```python
from build123d import *

# Parameters (mm, degrees)
SKETCH1_W                    = 98
SKETCH1_H                    = 32.71
BASE_FLANGE1_DEPTH           = 1.016
EDGE_FLANGE1_DEPTH           = 18
EDGE_FLANGE2_STRIP_CUT_DEPTH = 98
EDGE_FLANGE2_DEPTH           = 98
EDGE_FLANGE3_STRIP_CUT_DEPTH = 98
EDGE_FLANGE3_DEPTH           = 98
CUT_EXTRUDE1_REACH           = 115.066
SKETCH17_R                   = 1.1303


# Sheet-metal steps are written as plain solids
with BuildPart() as part:
    # Sketch1 → Base-Flange1 (new body)
    with BuildSketch(Plane.XY):
        with Locations((49, 16.355)):
            Rectangle(SKETCH1_W, SKETCH1_H)
        with BuildLine():
            Line((61.25, 18.71), (61.25, 3.21))
            ThreePointArc((61.25, 3.21), (61.542893219, 2.502893219), (62.25, 2.21))
            Line((62.25, 2.21), (70.25, 2.21))
            ThreePointArc((70.25, 2.21), (70.957106781, 2.502893219), (71.25, 3.21))
            Line((71.25, 3.21), (71.25, 6.21))
            ThreePointArc((71.25, 6.21), (71.542893219, 6.917106781), (72.25, 7.21))
            Line((72.25, 7.21), (82.25, 7.21))
            ThreePointArc((82.25, 7.21), (82.957106781, 7.502893219), (83.25, 8.21))
            Line((83.25, 8.21), (83.25, 29.21))
            ThreePointArc((83.25, 29.21), (82.957106781, 29.917106781), (82.25, 30.21))
            Line((82.25, 30.21), (72.25, 30.21))
            ThreePointArc((72.25, 30.21), (71.542893219, 29.917106781), (71.25, 29.21))
            Line((71.25, 29.21), (71.25, 20.71))
            ThreePointArc((71.25, 20.71), (70.957106781, 20.002893219), (70.25, 19.71))
            Line((70.25, 19.71), (62.25, 19.71))
            ThreePointArc((62.25, 19.71), (61.542893219, 19.417106781), (61.25, 18.71))
        make_face(mode=Mode.SUBTRACT)
        with BuildLine():
            Line((25.75, 30.21), (15.75, 30.21))
            ThreePointArc((15.75, 30.21), (15.042893219, 29.917106781), (14.75, 29.21))
            Line((14.75, 29.21), (14.75, 8.21))
            ThreePointArc((14.75, 8.21), (15.042893219, 7.502893219), (15.75, 7.21))
            Line((15.75, 7.21), (25.75, 7.21))
            ThreePointArc((25.75, 7.21), (26.457106781, 6.917106781), (26.75, 6.21))
            Line((26.75, 6.21), (26.75, 3.21))
            ThreePointArc((26.75, 3.21), (27.042893219, 2.502893219), (27.75, 2.21))
            Line((27.75, 2.21), (35.75, 2.21))
            ThreePointArc((35.75, 2.21), (36.457106781, 2.502893219), (36.75, 3.21))
            Line((36.75, 3.21), (36.75, 18.71))
            ThreePointArc((36.75, 18.71), (36.457106781, 19.417106781), (35.75, 19.71))
            Line((35.75, 19.71), (27.75, 19.71))
            ThreePointArc((27.75, 19.71), (27.042893219, 20.002893219), (26.75, 20.71))
            Line((26.75, 20.71), (26.75, 29.21))
            ThreePointArc((26.75, 29.21), (26.457106781, 29.917106781), (25.75, 30.21))
        make_face(mode=Mode.SUBTRACT)
    extrude(amount=-BASE_FLANGE1_DEPTH)

    # Edge-Flange1 section (across the edge) → Edge-Flange1 (add)
    with BuildSketch(Plane(origin=(40, 33.4466, -1.016), x_dir=(0, -1, 0), z_dir=(1, 0, 0))):
        with BuildLine():
            Line((-1.016, 0.7366), (-1.016, 17.984))
            Line((-1.016, 17.984), (0, 17.984))
            Line((0, 17.984), (0, 0.7366))
            ThreePointArc((0, 0.7366), (0.215745145, 0.215745145), (0.7366, 0))
            Line((0.7366, 0), (0.7366, -1.016))
            ThreePointArc((0.7366, -1.016), (-0.502675345, -0.502675345), (-1.016, 0.7366))
        make_face()
    extrude(amount=EDGE_FLANGE1_DEPTH)

    # Edge-Flange2 strip (across the edge) → Edge-Flange2 strip cut (cut)
    with BuildSketch(Plane(origin=(0, 0, 0), x_dir=(0, 0.8660254037844364, 0.5000000000000041), z_dir=(1, 0, 0))):
        Polygon((-4.935055866, 1.676080086), (-0.1397, -1.092519914), (0.3683, -0.212638104), (-4.427055866, 2.555961896), align=None)
    extrude(amount=EDGE_FLANGE2_STRIP_CUT_DEPTH, mode=Mode.SUBTRACT)

    # Edge-Flange2 section (across the edge) → Edge-Flange2 (add)
    with BuildSketch(Plane(origin=(0, 0, 0), x_dir=(0, 0.8660254037844364, 0.5000000000000041), z_dir=(1, 0, 0))):
        with BuildLine():
            Line((-1.016, 0.425276208), (-1.016, 14.163412127))
            Line((-1.016, 14.163412127), (0, 14.163412127))
            Line((0, 14.163412127), (0, 0.425276208))
            ThreePointArc((0, 0.425276208), (0.098685688, 0.056976208), (0.3683, -0.212638104))
            Line((0.3683, -0.212638104), (-0.1397, -1.092519914))
            ThreePointArc((-0.1397, -1.092519914), (-0.781196123, -0.451023792), (-1.016, 0.425276208))
        make_face()
    extrude(amount=EDGE_FLANGE2_DEPTH)

    # Edge-Flange3 strip (across the edge) → Edge-Flange3 strip cut (cut)
    with BuildSketch(Plane(origin=(0, -7.081706063, 12.265874706), x_dir=(0, 1, 0), z_dir=(1, 0, 0))):
        Polygon((-3.549796123, 4.116427241), (-0.781196123, -0.678928625), (0.098685688, -0.170928625), (-2.669914312, 4.624427241), align=None)
    extrude(amount=EDGE_FLANGE3_STRIP_CUT_DEPTH, mode=Mode.SUBTRACT)

    # Edge-Flange3 section (across the edge) → Edge-Flange3 (add)
    with BuildSketch(Plane(origin=(0, -7.081706063, 12.265874706), x_dir=(0, 1, 0), z_dir=(1, 0, 0))):
        with BuildLine():
            Line((-1.016, 0.197371375), (-1.016, 24.72776362))
            Line((-1.016, 24.72776362), (0, 24.72776362))
            Line((0, 24.72776362), (0, 0.197371375))
            ThreePointArc((0, 0.197371375), (0.025099036, 0.006725267), (0.098685688, -0.170928625))
            Line((0.098685688, -0.170928625), (-0.781196123, -0.678928625))
            ThreePointArc((-0.781196123, -0.678928625), (-0.956281603, -0.256234883), (-1.016, 0.197371375))
        make_face()
    extrude(amount=EDGE_FLANGE3_DEPTH)

    # Sketch17 → Cut-Extrude1 (cut, up to next)
    with BuildSketch(Plane(origin=(0, 34.4626, 0), x_dir=(1, 0, 0), z_dir=(0, 1, 0)), mode=Mode.PRIVATE) as cut_extrude1_sk1:
        with Locations(Location((54, 10, 0), (0, 0, 270))):
            Circle(SKETCH17_R)
    cut_extrude1_tool1 = extrude(cut_extrude1_sk1.sketch, amount=-CUT_EXTRUDE1_REACH, mode=Mode.PRIVATE) & part.part
    # Sketch17 → Cut-Extrude1 (cut, up to next)
    with BuildSketch(Plane(origin=(0, 34.4626, 0), x_dir=(1, 0, 0), z_dir=(0, 1, 0)), mode=Mode.PRIVATE) as cut_extrude1_sk2:
        with Locations(Location((54, 16, 0), (0, 0, 270))):
            Circle(SKETCH17_R)
    cut_extrude1_tool2 = extrude(cut_extrude1_sk2.sketch, amount=-CUT_EXTRUDE1_REACH, mode=Mode.PRIVATE) & part.part
    # Sketch17 → Cut-Extrude1 (cut, up to next)
    with BuildSketch(Plane(origin=(0, 34.4626, 0), x_dir=(1, 0, 0), z_dir=(0, 1, 0)), mode=Mode.PRIVATE) as cut_extrude1_sk3:
        with Locations(Location((44, 10, 0), (0, 0, 270))):
            Circle(SKETCH17_R)
    cut_extrude1_tool3 = extrude(cut_extrude1_sk3.sketch, amount=-CUT_EXTRUDE1_REACH, mode=Mode.PRIVATE) & part.part
    # Sketch17 → Cut-Extrude1 (cut, up to next)
    with BuildSketch(Plane(origin=(0, 34.4626, 0), x_dir=(1, 0, 0), z_dir=(0, 1, 0)), mode=Mode.PRIVATE) as cut_extrude1_sk4:
        with Locations(Location((44, 16, 0), (0, 0, 270))):
            Circle(SKETCH17_R)
    cut_extrude1_tool4 = extrude(cut_extrude1_sk4.sketch, amount=-CUT_EXTRUDE1_REACH, mode=Mode.PRIVATE) & part.part
    add(cut_extrude1_tool1.solids().sort_by_distance((54, 34.4626, -10))[0], mode=Mode.SUBTRACT)
    add(cut_extrude1_tool2.solids().sort_by_distance((54, 34.4626, -16))[0], mode=Mode.SUBTRACT)
    add(cut_extrude1_tool3.solids().sort_by_distance((44, 34.4626, -10))[0], mode=Mode.SUBTRACT)
    add(cut_extrude1_tool4.solids().sort_by_distance((44, 34.4626, -16))[0], mode=Mode.SUBTRACT)


solid = part.part
```
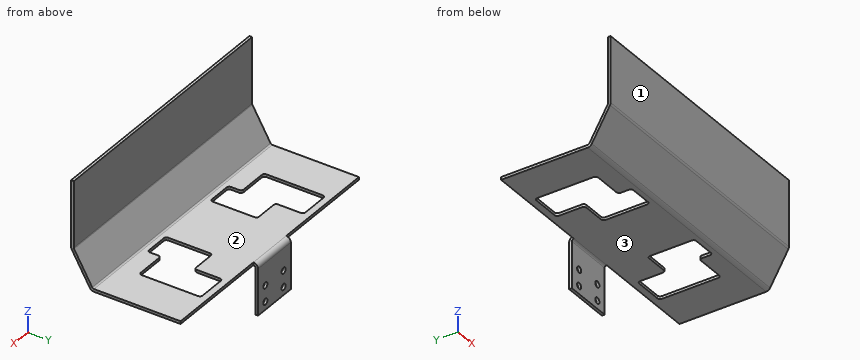
Part model, mm, in its own coordinate system. Face numbers are marked on the shaded views. A direction names the side the tool comes from. Coordinates: 2 decimals unless noted, no trailing zeros. Write each loop counter-clockwise with the first axis right and the second up, starting at its lowest first coordinate (ties: lowest second). Pieces come first, ordered by that corner, then holes.
Item 1: Slice it at C-C (y = 12.5). Write the cut outline in (x, z).
Item 2: Probe line 1 (X direction, y = 33.9, z = -10); line 2 (Z direction, x = 58, y = 32.5); line 3 (Y direction, x = 44, z = 21.5). List the from-to ranges inside material, lowest first.
Item 3: Which spindle directions (+Z, -Z, +X, -X, +Y, -Y) get a long thin tool onto all of the face, cutting with end or side? Do the marked faces 1, 2 and 3. Say none if no direction does.
Item 4: Slice it at A-A (x = 54). Write the cut outline in (y, z).
Item 5: Slice it at D-D (x = 76.5). Write the cut outline in (y, z), and give its area (3 significant figures).
Item 6: Slice it at B-B (z = -16). Write the cut outline in (x, y), and give its area (3 significant figures).
Item 7: Pin check, flat tips, straight feed: pin 1 (1.5 mm diameter, centred on x = 47, y = 8.5, fed in from -Z); pin 2 (4 mm diameter, centred on x = 63.5, y = 22.5, fed in from +Z); pin 3 (1.1 mm diameter, centred on x = 32, z = -0.5, fed in from -Y). Stop position of each tip, or through.
Results found:
1. outline: (0, -1.02) - (14.75, -1.02) - (14.75, 0) - (0, 0) - close; (36.75, -1.02) - (61.25, -1.02) - (61.25, 0) - (36.75, 0) - close; (83.25, -1.02) - (98, -1.02) - (98, 0) - (83.25, 0) - close
2. line 1: x = 40 to 42.87, 45.13 to 52.87, 55.13 to 58
2. line 2: z = -1.02 to 0
2. line 3: y = -8.1 to -7.08
3. face 1: +Z, -Z, +X, -X, -Y
3. face 2: +Z, +X, -X, +Y
3. face 3: -Z, +X, -X, -Y
4. outline: (-8.1, 12.46) arc R1.75 ccw to (-7.86, 11.59) - (-1.09, -0.14) arc R1.75 ccw to (0.43, -1.02) - (32.71, -1.02) arc R0.74 cw to (33.45, -1.75) - (33.45, -8.87) - (34.46, -8.87) - (34.46, -1.75) arc R1.75 ccw to (32.71, 0) - (0.43, 0) arc R0.74 cw to (-0.21, 0.37) - (-6.98, 12.09) arc R0.74 cw to (-7.08, 12.46) - (-7.08, 36.99) - (-8.1, 36.99) - close; (33.45, -19) - (34.46, -19) - (34.46, -17.13) - (33.45, -17.13) - close; (33.45, -14.87) - (34.46, -14.87) - (34.46, -11.13) - (33.45, -11.13) - close
5. outline: (-8.1, 12.46) arc R1.75 ccw to (-7.86, 11.59) - (-1.09, -0.14) arc R1.75 ccw to (0.43, -1.02) - (7.21, -1.02) - (7.21, 0) - (0.43, 0) arc R0.74 cw to (-0.21, 0.37) - (-6.98, 12.09) arc R0.74 cw to (-7.08, 12.46) - (-7.08, 36.99) - (-8.1, 36.99) - close; (30.21, -1.02) - (32.71, -1.02) - (32.71, 0) - (30.21, 0) - close
5. area: 50.1 mm2
6. outline: (40, 33.45) - (42.87, 33.45) - (42.87, 34.46) - (40, 34.46) - close; (45.13, 33.45) - (52.87, 33.45) - (52.87, 34.46) - (45.13, 34.46) - close; (55.13, 33.45) - (58, 33.45) - (58, 34.46) - (55.13, 34.46) - close
6. area: 13.7 mm2
7. pin 1: stops at z = -1.02
7. pin 2: stops at z = 0
7. pin 3: stops at y = -1.2
